```python
from build123d import *


with BuildPart() as f1:
    # F0 (on Front) → F1 (revolve)
    with BuildSketch(Plane.XZ):
        with BuildLine():
            Line((259.395182, 0), (0, 0))
            Line((0, 0), (0, -3.429))
            Line((0, -3.429), (260.757632, -3.429))
            Line((260.757632, -3.429), (268.478561, -12.634282))
            ThreePointArc((268.478561, -12.634282), (271.837306, -15.21236), (275.971, -16.129))
            Line((275.971, -16.129), (295.021, -16.129))
            Line((295.021, -16.129), (295.021, -12.7))
            Line((295.021, -12.7), (275.971, -12.7))
            ThreePointArc((275.971, -12.7), (273.286783, -12.104779), (271.10578, -10.430703))
            Line((271.10578, -10.430703), (264.260402, -2.269297))
            ThreePointArc((264.260402, -2.269297), (262.079399, -0.595221), (259.395182, 0))
        make_face()
    revolve(axis=Axis((0, 0, -1.7145), (0, 0, -1)))


solid = f1.part
```
Geometry check sheet. Reference: the model listing, model coordinates, mm. A direction names the side the tool comes from. Round coordinates to 2 decimals unless told otherwise and drop trailing zeros. Order: outer loops, then holes, each group sorted by start corner. A loop starts at its lowest first (then second) coordinate and runs counter-clockwise, first axis right, second up. Notation, with made-up numbers: (72, 60) - (106, 60) arc R21 ccw to (106, 81) - close; hole circle Ø1 at (59, 1). An arc over 180 degrees is marked (long way). Use a Markdown table: item, result. Add a question column.
(1) Material ranges on line 1 along Z through (x, y) = (240, -36.5); line 2 along Y through (x, z) = (-184.5, -11); line 3 along X through (y, z) = (193, -8), recorded low to high. Write a range as [from, to].
(2) Sectioned sample at C-C, the plane z = -6. Enter the section's corners in (x, y).
(3) Sectioned sample at A-A, the plane x = 0. Enter the section's corners in (y, z).
(4) Depth check by flat-ended pin: pin 1 (5 mm diameter, centred on y = 112, z = -14, fed in from +X); pin 2 (1.5 mm diameter, centred on y = -26, z = -2.5, fed in from -X); pin 3 (5 mm diameter, centred on x = 0, z = -6, fed in from +Y). Enter the tip coordinate at first touch or a pass-through.
(5) Tool access check on faces 1 (the flat face through (195.3, 195.3, -12.7)), 2 (the flat face through (-195.3, 195.3, -16.129)). Record the directions out of +Z, -Z, +X, -X, +Y, -Y that give a thin tool (end or side, any length) a straight path to the whole face; none if there is none.
(6) Release check for a two-part mould opening along X. For faces 3 (the cylindrical face through (-63.955, 288.006, -14.39)), 4 (the flat face through (4, -4, -3.429)), 5 (the flat face through (-4, -4, 0)) record: pulls with the +X half, pulls with the -X half, needs draft (parallel to the pull), parting line crosses it, or undercut.
Answers below:
| question | item | result |
|---|---|---|
| 1 | line 1 | [-3.43, 0] |
| 1 | line 2 | [-199.38, -193.15], [193.15, 199.38] |
| 1 | line 3 | [-187.48, -181], [181, 187.48] |
| 2 | outline | circle Ø534.78 at (0, 0); hole circle Ø525.83 at (0, 0) |
| 3 | outline | (-295.02, -16.13) - (-275.97, -16.13) arc R9.78 ccw to (-268.48, -12.63) - (-260.76, -3.43) - (260.76, -3.43) - (268.48, -12.63) arc R9.78 ccw to (275.97, -16.13) - (295.02, -16.13) - (295.02, -12.7) - (275.97, -12.7) arc R6.35 cw to (271.11, -10.43) - (264.26, -2.27) arc R6.35 ccw to (259.4, 0) - (-259.4, 0) arc R6.35 ccw to (-264.26, -2.27) - (-271.11, -10.43) arc R6.35 cw to (-275.97, -12.7) - (-295.02, -12.7) - close |
| 4 | pin 1 | x = 273.95 |
| 4 | pin 2 | x = -263.81 |
| 4 | pin 3 | y = 269.49 |
| 5 | face 1 | +Z |
| 5 | face 2 | -Z, +X, -X, +Y, -Y |
| 6 | face 3 | parting line crosses it |
| 6 | face 4 | undercut |
| 6 | face 5 | needs draft |
